Part model, mm, in its own coordinate system. Round coordinates to 2 decimals unless told otherwise and drop trailing zeros. Write each loop counter-clockwise with the first axis right and the second up, starting at its lowest first coordinate (ties: lowest second). Pieces come first, ordered by that corner, then holes. Notation, with made-up numbers: M 62.25,32 L 68.25,32 A15 ccw 68.25,54 Z; hole C 49,87 d2. An arc over 180 degrees is marked long. Answer as a JSON object with one key per item and string values. Group by question number.
1. Band-saw the part on A-A, the plane x = 40. Write the cut outline in (y, z).
2. Band-saw the part on B-B, the plane x = -27.5. Write the cut outline in (y, z).
3. Drill centre lines: line 1 (Y direction, x = 40, z = 2); line 2 (Z direction, x = -9.5, y = -0.25); line 3 (X direction, y = 0.25, z = -35.5). Where is each one in solid material? Low to high. Write a range as from..to.
4. Drop a flat-ended pin along its axis: pin 1 (1 mm diameter, centred on x = 34.5, y = 1.5, fed in from -Z). Give the stop position or say it passes through.
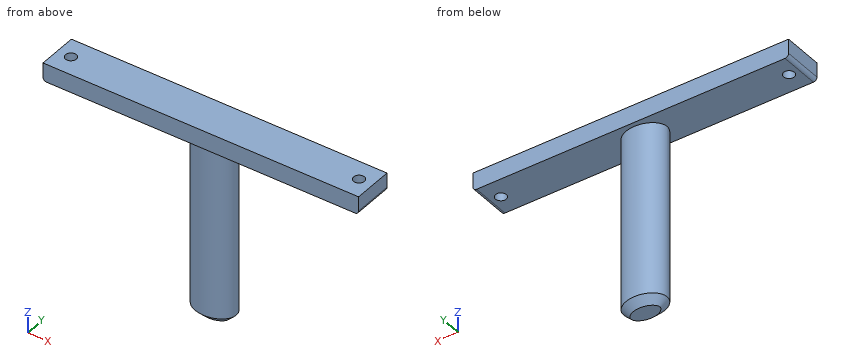
Autodesk Inventor part; units mm, degrees
ref_plane "YZ Plane" through (0, 0, 0) normal (1, 0, 0) x (0, 1, 0)
ref_plane "XZ Plane" through (0, 0, 0) normal (0, 1, 0) x (-1, 0, 0)
ref_plane "XY Plane" through (0, 0, 0) normal (0, 0, 1) x (1, 0, 0)
sketch "Sketch1" plane through (0, 0, 0) normal (0, 0, 1) x (1, 0, 0)
  line L0 (-40, 0) -> (40, 0)
  circle A0 centre (-40, 0) radius 1.5
  circle A1 centre (40, 0) radius 1.5
  line L1 (-43.8161, 5.5412) -> (43.8161, 5.5412)
  line L2 (43.8161, 5.5412) -> (43.8161, -5.5412)
  line L3 (43.8161, -5.5412) -> (-43.8161, -5.5412)
  line L4 (-43.8161, -5.5412) -> (-43.8161, 5.5412)
  ellipse E0 centre (-0.0839, -0.042) end of major axis (-6.111, -0.042) minor radius 4.3359
  point P0 (0, 0)
  point P1 (0, 0)
  point P2 (0, -5.5412)
  point P3 (-43.8161, 0)
  point P4 (43.8161, 0)
extrude "Extrusion2" add sketch "Sketch1" along normal blind 5
sketch "Sketch4" plane through (0, 0, 0) normal (0, 0, -1) x (-1, 0, 0)
  ellipse E0 centre (0.0839, -0.042) end of major axis (-5.9431, -0.042) minor radius 4.3359
  point P0 (0, 0)
extrude "Extrusion3" add sketch "Sketch4" along normal blind 50 and the other way blind 5
chamfer "Chamfer1" distance 2 angle 45 1 edges at (-6.111, -0.042, -50)
fillet "Fillet1" radius 1 1 edges at (-43.8161, 0, 0)
fillet "Fillet2" radius 1 1 edges at (43.8161, 0, 0)
properties part number "apoioG"
Worked answers:
{
 "1": {"outline": "M -5.54,0 L -1.5,0 L -1.5,5 L -5.54,5 Z; M 1.5,0 L 5.54,0 L 5.54,5 L 1.5,5 Z"},
 "2": {"outline": "M -5.54,0 L 5.54,0 L 5.54,5 L -5.54,5 Z"},
 "3": {"line 1": "y = -5.54..-1.5, 1.5..5.54", "line 2": "z = 0..5", "line 3": "x = -6.1..5.93"},
 "4": {"pin 1": "stops at z = 0"}
}
